from build123d import *

# Parameters (mm, degrees)
BOSS_EXTRUDE1_DEPTH = 8
SKETCH2_R           = 1.651
CUT_EXTRUDE1_DEPTH  = 63.737548565
SKETCH3_R           = 4
CUT_EXTRUDE2_DEPTH  = 4
BOSS_EXTRUDE2_DEPTH = 12.1
BOSS_EXTRUDE3_DEPTH = 4
SKETCH6_R           = 1.1
CUT_EXTRUDE4_DEPTH  = 4
SKETCH7_W           = 1.6764
SKETCH7_H           = 4.7752
CUT_EXTRUDE5_DEPTH  = 89.164959026
SKETCH8_W           = 48
SKETCH8_H           = 2.725
BOSS_EXTRUDE4_DEPTH = 64
SKETCH9_W           = 48
SKETCH9_H           = 72
BOSS_EXTRUDE5_DEPTH = 6
SKETCH10_R          = 28
CUT_EXTRUDE6_DEPTH  = 2
SKETCH12_R          = 4
CUT_EXTRUDE7_DEPTH  = 126.778478386
SKETCH13_W          = 6
SKETCH13_H          = 14.4
CUT_EXTRUDE8_DEPTH  = 99.081598682


with BuildPart() as part:
    # Sketch1 → Boss-Extrude1 (new body)
    with BuildSketch(Plane(origin=(0, 0, 0), x_dir=(1, 0, 0), z_dir=(0, 1, 0))):
        with BuildLine():
            Line((-44, 28), (-36, 28))
            ThreePointArc((-36, 28), (-33.878679656, 27.121320344), (-33, 25))
            Line((-33, 25), (-33, 19))
            ThreePointArc((-33, 19), (-33.878679656, 16.878679656), (-36, 16))
            Line((-36, 16), (-44, 16))
            Line((-44, 16), (-44, -16))
            Line((-44, -16), (-36, -16))
            ThreePointArc((-36, -16), (-33.878679656, -16.878679656), (-33, -19))
            Line((-33, -19), (-33, -25))
            ThreePointArc((-33, -25), (-33.878679656, -27.121320344), (-36, -28))
            Line((-36, -28), (-44, -28))
            Line((-44, -28), (-44, -44))
            Line((-44, -44), (44, -44))
            Line((44, -44), (44, -28))
            Line((44, -28), (36, -28))
            ThreePointArc((36, -28), (33.878679656, -27.121320344), (33, -25))
            Line((33, -25), (33, -19))
            ThreePointArc((33, -19), (33.878679656, -16.878679656), (36, -16))
            Line((36, -16), (44, -16))
            Line((44, -16), (44, 16))
            Line((44, 16), (36, 16))
            ThreePointArc((36, 16), (33.878679656, 16.878679656), (33, 19))
            Line((33, 19), (33, 25))
            ThreePointArc((33, 25), (33.878679656, 27.121320344), (36, 28))
            Line((36, 28), (44, 28))
            Line((44, 28), (44, 44))
            Line((44, 44), (-44, 44))
            Line((-44, 44), (-44, 28))
        make_face()
    extrude(amount=BOSS_EXTRUDE1_DEPTH)

    # Sketch2 → Cut-Extrude1 (cut, through all)
    with BuildSketch(Plane(origin=(0, 8, 0), x_dir=(1, 0, 0), z_dir=(0, 1, 0))):
        with Locations(Location((-36, 36, 0), (0, 0, 270))):
            Circle(SKETCH2_R)
        with Locations(Location((36, 36, 0), (0, 0, 90))):
            Circle(SKETCH2_R)
        with Locations(Location((36, -36, 0), (0, 0, 270))):
            Circle(SKETCH2_R)
        with Locations(Location((-36, -36, 0), (0, 0, 90))):
            Circle(SKETCH2_R)
    extrude(amount=-CUT_EXTRUDE1_DEPTH, mode=Mode.SUBTRACT)

    # Sketch3 → Cut-Extrude2 (cut)
    with BuildSketch(Plane(origin=(0, 8, 0), x_dir=(1, 0, 0), z_dir=(0, 1, 0))):
        with Locations(Location((-36, 36, 0), (0, 0, 270))):
            Circle(SKETCH3_R)
        with Locations(Location((36, 36, 0), (0, 0, 270))):
            Circle(SKETCH3_R)
        with Locations(Location((36, -36, 0), (0, 0, 270))):
            Circle(SKETCH3_R)
        with Locations(Location((-36, -36, 0), (0, 0, 270))):
            Circle(SKETCH3_R)
    extrude(amount=-CUT_EXTRUDE2_DEPTH, mode=Mode.SUBTRACT)

    # Sketch4 → Boss-Extrude2 (add)
    with BuildSketch(Plane(origin=(0, 8, 0), x_dir=(1, 0, 0), z_dir=(0, 1, 0))):
        Polygon((0, -12.5), (3, -12.5), (3, -30.7), (25.5, -30.7), (25.5, -12.5), (28.5, -12.5), (34.1, -12.5), (34.1, -16.5), (28.5, -16.5), (28.5, -33.7), (0, -33.7), (0, -16.5), (-5.6, -16.5), (-5.6, -12.5), align=None)
    extrude(amount=BOSS_EXTRUDE2_DEPTH)

    # Sketch5 → Boss-Extrude3 (add)
    with BuildSketch(Plane(origin=(0, 20.1, 0), x_dir=(1, 0, 0), z_dir=(0, 1, 0))):
        Polygon((3, -12.5), (25.5, -12.5), (34.1, -12.5), (34.1, -16.5), (28.5, -16.5), (28.5, -33.7), (0, -33.7), (0, -16.5), (-5.6, -16.5), (-5.6, -12.5), align=None)
    extrude(amount=BOSS_EXTRUDE3_DEPTH)

    # Sketch6 → Cut-Extrude4 (cut)
    with BuildSketch(Plane(origin=(0, 0, 12.5), x_dir=(-1, 0, 0), z_dir=(0, 0, -1))):
        with Locations((-28.1, 14.05)):
            Circle(SKETCH6_R)
        with Locations((-0.4, 14.05)):
            Circle(SKETCH6_R)
    extrude(amount=-CUT_EXTRUDE4_DEPTH, mode=Mode.SUBTRACT)

    # Sketch7 → Cut-Extrude5 (cut, through all)
    with BuildSketch(Plane(origin=(28.5, 0, 0), x_dir=(0, 0, -1), z_dir=(1, 0, 0))):
        with Locations((-17.3382, 14.05)):
            Rectangle(SKETCH7_W, SKETCH7_H)
    extrude(amount=-CUT_EXTRUDE5_DEPTH, mode=Mode.SUBTRACT)

    # Sketch8 → Boss-Extrude4 (add)
    with BuildSketch(Plane(origin=(0, 8, 0), x_dir=(1, 0, 0), z_dir=(0, 1, 0))):
        with Locations((0, 42.6375)):
            Rectangle(SKETCH8_W, SKETCH8_H)
        with Locations((0, -42.6375)):
            Rectangle(SKETCH8_W, SKETCH8_H)
    extrude(amount=BOSS_EXTRUDE4_DEPTH)

    # Sketch9 → Boss-Extrude5 (add)
    with BuildSketch(Plane.XY.offset(44)):
        with Locations((0, 36)):
            Rectangle(SKETCH9_W, SKETCH9_H)
    boss_extrude5 = extrude(amount=BOSS_EXTRUDE5_DEPTH)

    # Mirror1: Boss-Extrude5 across plane
    add(boss_extrude5.mirror(Plane.XY))

    # Sketch10 → Cut-Extrude6 (cut)
    with BuildSketch(Plane(origin=(0, 0, 41.275), x_dir=(-1, 0, 0), z_dir=(0, 0, -1))):
        with Locations((0, 48)):
            Circle(SKETCH10_R)
    cut_extrude6 = extrude(amount=-CUT_EXTRUDE6_DEPTH, mode=Mode.SUBTRACT)

    # Sketch12 → Cut-Extrude7 (cut, through all)
    with BuildSketch(Plane(origin=(0, 0, 43.275), x_dir=(-1, 0, 0), z_dir=(0, 0, -1))):
        with Locations((0, 48)):
            Circle(SKETCH12_R)
    cut_extrude7 = extrude(amount=-CUT_EXTRUDE7_DEPTH, mode=Mode.SUBTRACT)

    # Mirror2: Cut-Extrude6, Cut-Extrude7 across plane
    add(cut_extrude6.mirror(Plane.XY), mode=Mode.SUBTRACT)
    add(cut_extrude7.mirror(Plane.XY), mode=Mode.SUBTRACT)

    # Sketch13 → Cut-Extrude8 (cut, through all)
    with BuildSketch(Plane.XZ):
        with Locations((-23, -30.8)):
            Rectangle(SKETCH13_W, SKETCH13_H)
    extrude(amount=-CUT_EXTRUDE8_DEPTH, mode=Mode.SUBTRACT)


solid = part.part
For this review, take the finished solid that the model builds, in its own axes (mm). A direction names the side the tool comes from. Coordinates: 2 decimals unless noted, no trailing zeros. Write each loop counter-clockwise with the first axis right and the second up, starting at its lowest first coordinate (ties: lowest second). Pieces come first, ordered by that corner, then holes. Notation, with made-up numbers: (62, -18) -> (107, -18) arc R25 ccw to (107, 2) -> close; hole circle Ø10 at (22.5, 15.5). An arc over 180 degrees is marked (long way). Write each question's results on one line, items separated by ' | '. Start each with the question number.
1) Consider section A-A (y = 59.5). Write out the cut boundary in (x, z) (3 decimals), plus the area to 3 significant figures.
2) Consider section B-B (y = 48). Write out the cut boundary in (x, z) (3 decimals).
3) Wall thickness on L1, parallel to X at y = 1.95, z = -36; L2, parallel to X at y = 2.5, z = 36; L3, parallel to Y at x = 15, z = 25: over which ranges is each line inside the solid? List them lowest first. Write a range as [from, to].
4) Consider section C-C (x = 10). Write out the cut boundary in (y, z) (3 decimals).
5) Consider section D-D (z = -22). Write out the cut boundary in (x, y).
6) Insertion check: pin 1 (2.5 mm diameter, centred on y = 38.5, z = 46.5, fed in from -X); pin 2 (4 mm diameter, centred on x = -21.5, z = 4.5, fed in from +Y); pin 3 (5 mm diameter, centred on x = -31, z = -20.5, fed in from -Y); pin 4 (4 mm diameter, centred on x = -38, y = 2.5, fed in from +Z). Each pin has a flat end and moves straight along its axis. Give the tip position at first contact, or say it passes through.
7) The part is to be moulded in two halves that separate along Z. For faces 1 (the face through (-36, 4, -34)), 2 (the face through (44, 4, -36)), say which applies: +Z half, -Z half, draft (parallel to the pull), parting line (faces both ways), or undercut.
8) For faces 3 (the face through (-21, 69, 41.275)), 4 (the face through (-20, 4, -31)), 5 (the face through (-40, 4, -28)), 6 (the face through (31, 16, 16.5)), list the 3-axis set-ups (+Z, -Z, +X, -X, +Y, -Y) from which the entire face can be reached by the end or side of a thin tool; tool diameter is ignored.
Geometry says:
1) outline: (-24, -50) -> (24, -50) -> (24, -43.275) -> (-24, -43.275) -> close; (-24, 43.275) -> (24, 43.275) -> (24, 50) -> (-24, 50) -> close | area: 646 mm^2
2) outline: (-24, -50) -> (-4, -50) -> (-4, -43.275) -> (-24, -43.275) -> close; (-24, 43.275) -> (-4, 43.275) -> (-4, 50) -> (-24, 50) -> close; (4, -50) -> (24, -50) -> (24, -43.275) -> (4, -43.275) -> close; (4, 43.275) -> (24, 43.275) -> (24, 50) -> (4, 50) -> close
3) L1: [-44, -37.65], [-34.35, -26], [-20, 34.35], [37.65, 44] | L2: [-44, -37.65], [-34.35, 34.35], [37.65, 44] | L3: [0, 8], [20.1, 24.1]
4) outline: (0, -50) -> (72, -50) -> (72, -43.275) -> (21.847, -43.275) -> (21.847, -41.275) -> (8, -41.275) -> (8, 30.7) -> (20.1, 30.7) -> (20.1, 12.5) -> (24.1, 12.5) -> (24.1, 33.7) -> (8, 33.7) -> (8, 41.275) -> (21.847, 41.275) -> (21.847, 43.275) -> (72, 43.275) -> (72, 50) -> (0, 50) -> close
5) outline: (-33, 0) -> (33, 0) -> (33, 8) -> (-33, 8) -> close
6) pin 1: x = -24 | pin 2: y = 8 | pin 3: y = 0 | pin 4: z = 44
7) face 1: undercut | face 2: draft
8) face 3: +X, -X, +Y | face 4: +Y, -Y | face 5: -X, +Y, -Y | face 6: +X
